Read the model definition and answer for the solid it produces. Units are mm, in the model's axes. A direction names the side the tool comes from. Round coordinates to 2 decimals unless told otherwise and drop trailing zeros. Write each loop counter-clockwise with the first axis right and the second up, starting at its lowest first coordinate (ties: lowest second). Pieces come first, ordered by that corner, then holes.
from build123d import *

# Parameters (mm, degrees)
SKETCH1_W           = 280
SKETCH1_H           = 210
BOSS_EXTRUDE1_DEPTH = 15
SKETCH2_R           = 5
BOSS_EXTRUDE2_DEPTH = 50
SKETCH3_W           = 10
SKETCH3_H           = 30
BOSS_EXTRUDE3_DEPTH = 50
SKETCH4_R           = 13
CUT_EXTRUDE1_DEPTH  = 20
SKETCH5_W           = 360.4909063
SKETCH5_H           = 249.182613404
SKETCH5_W_2         = 248.173776912
SKETCH5_H_2         = 125.095724948
CUT_EXTRUDE5_DEPTH  = 15
CUT_EXTRUDE6_START  = -65
SKETCH7_R           = 5
CUT_EXTRUDE6_DEPTH  = 65
SKETCH8_R           = 10.1
CUT_EXTRUDE11_DEPTH = 12
SKETCH13_W          = 26.98462743
SKETCH13_H          = 41.59552633
CUT_EXTRUDE12_DEPTH = 148.681383345
SKETCH11_W          = 17.231524428
SKETCH11_H          = 37.334969593
CUT_EXTRUDE13_DEPTH = 50
CUT_EXTRUDE16_DEPTH = 140.766916639
SKETCH16_R          = 13
CUT_EXTRUDE20_DEPTH = 5
CUT_EXTRUDE22_DEPTH = 2
SKETCH18_R          = 15.15
CUT_EXTRUDE23_DEPTH = 2
SKETCH9_W           = 29.33
SKETCH9_H           = 16.92
CUT_EXTRUDE24_DEPTH = 140.766916639


with BuildPart() as part:
    # Sketch1 → Boss-Extrude1 (new body)
    with BuildSketch(Plane(origin=(0, 0, 0), x_dir=(1, 0, 0), z_dir=(0, 1, 0))):
        Rectangle(SKETCH1_W, SKETCH1_H)
    extrude(amount=BOSS_EXTRUDE1_DEPTH)

    # Sketch2 → Boss-Extrude2 (add)
    with BuildSketch(Plane(origin=(0, 15, 0), x_dir=(1, 0, 0), z_dir=(0, 1, 0))):
        with Locations(Location((-100, 0, 0), (0, 0, 270))):
            Circle(SKETCH2_R)
        with Locations(Location((-100, 45, 0), (0, 0, 270))):
            Circle(SKETCH2_R)
        with Locations(Location((-100, -45, 0), (0, 0, 270))):
            Circle(SKETCH2_R)
    extrude(amount=BOSS_EXTRUDE2_DEPTH)

    # Sketch3 → Boss-Extrude3 (add)
    with BuildSketch(Plane(origin=(0, 15, 0), x_dir=(1, 0, 0), z_dir=(0, 1, 0))):
        Rectangle(SKETCH3_W, SKETCH3_H)
    extrude(amount=BOSS_EXTRUDE3_DEPTH)

    # Sketch4 → Cut-Extrude1 (cut)
    with BuildSketch(Plane(origin=(5, 0, 0), x_dir=(0, 0, -1), z_dir=(1, 0, 0))):
        with Locations((0, 41.236240869)):
            Circle(SKETCH4_R)
    extrude(amount=-CUT_EXTRUDE1_DEPTH, mode=Mode.SUBTRACT)

    # Sketch5 → Cut-Extrude5 (cut)
    with BuildSketch(Plane(origin=(0, 0, 0), x_dir=(1, 0, 0), z_dir=(0, 1, 0))):
        with Locations((1.345115322, -3.19464889)):
            Rectangle(SKETCH5_W, SKETCH5_H)
        Rectangle(SKETCH5_W_2, SKETCH5_H_2, mode=Mode.SUBTRACT)
    extrude(amount=CUT_EXTRUDE5_DEPTH, mode=Mode.SUBTRACT)

    # Sketch7 → Cut-Extrude6 (cut)
    with BuildSketch(Plane(origin=(0, 65, 0), x_dir=(1, 0, 0), z_dir=(0, 1, 0)).offset(CUT_EXTRUDE6_START)):
        with Locations(Location((-100, 45, 0), (0, 0, 270))):
            Circle(SKETCH7_R)
        with Locations(Location((-100, 0, 0), (0, 0, 270))):
            Circle(SKETCH7_R)
        with Locations(Location((-100, -45, 0), (0, 0, 270))):
            Circle(SKETCH7_R)
    extrude(amount=CUT_EXTRUDE6_DEPTH, mode=Mode.SUBTRACT)

    # Sketch8 → Cut-Extrude11 (cut)
    with BuildSketch(Plane.XZ):
        with Locations(Location((-100, 45, 0), (0, 0, 270))):
            Circle(SKETCH8_R)
        with Locations(Location((-100, 0, 0), (0, 0, 270))):
            Circle(SKETCH8_R)
        with Locations(Location((-100, -45, 0), (0, 0, 270))):
            Circle(SKETCH8_R)
    extrude(amount=-CUT_EXTRUDE11_DEPTH, mode=Mode.SUBTRACT)

    # Sketch13 → Cut-Extrude12 (cut, through all)
    with BuildSketch(Plane(origin=(0, 15, 0), x_dir=(1, 0, 0), z_dir=(0, 1, 0))):
        with Locations((-56.507686285, 0.099999998)):
            Rectangle(SKETCH13_W, SKETCH13_H)
    extrude(amount=-CUT_EXTRUDE12_DEPTH, mode=Mode.SUBTRACT)

    # Sketch11 → Cut-Extrude13 (cut)
    with BuildSketch(Plane(origin=(0, 65, 0), x_dir=(1, 0, 0), z_dir=(0, 1, 0))):
        with Locations((-3.002833284, 0.13632265)):
            Rectangle(SKETCH11_W, SKETCH11_H)
    extrude(amount=-CUT_EXTRUDE13_DEPTH, mode=Mode.SUBTRACT)

    # Sketch10 → Cut-Extrude16 (cut, through all)
    with BuildSketch(Plane(origin=(0, 15, 0), x_dir=(1, 0, 0), z_dir=(0, 1, 0))):
        Polygon((10.617962241, 13.651558309), (10.617962241, -16.40773575), (21.11227659, -7.629229077), (21.11227659, -32.023722987), (10.617962241, -26.348441691), (10.617962241, -56.40773575), (21.11227659, -47.629229077), (21.11227659, -62.347862477), (41.181983769, -80.61345612), (118.859305744, -85.146591928), (147.57727439, -51.586107965), (147.57727439, 65.118065893), (115.028872781, 75.532398006), (21.11227659, 80.76325418), (21.11227659, 62.347862473), (21.11227659, 47.976277013), (10.617962241, 53.651558309), (10.617962241, 23.59226425), (21.11227659, 32.370770923), (21.11227659, 7.976277013), align=None)
    extrude(amount=-CUT_EXTRUDE16_DEPTH, mode=Mode.SUBTRACT)

    # Sketch16 → Cut-Extrude20 (cut)
    with BuildSketch(Plane(origin=(0, 15, 0), x_dir=(1, 0, 0), z_dir=(0, 1, 0))):
        with Locations(Location((-100, 0, 0), (0, 0, 270))):
            Circle(SKETCH16_R)
    extrude(amount=-CUT_EXTRUDE20_DEPTH, mode=Mode.SUBTRACT)

    # Sketch17 → Cut-Extrude22 (cut)
    with BuildSketch(Plane.XZ):
        Polygon((-99.150124323, 10.064179616), (-99.150124323, 12.064179616), (-100.650124323, 12.064179616), (-100.650124323, 10.064179616), (-100.726397945, 9.213176312), (-99.150124323, 9.422776077), align=None)
    extrude(amount=-CUT_EXTRUDE22_DEPTH, mode=Mode.SUBTRACT)

    # Sketch18 → Cut-Extrude23 (cut)
    with BuildSketch(Plane(origin=(0, 15, 0), x_dir=(1, 0, 0), z_dir=(0, 1, 0))):
        with Locations(Location((-100, 0, 0), (0, 0, 270))):
            Circle(SKETCH18_R)
    extrude(amount=-CUT_EXTRUDE23_DEPTH, mode=Mode.SUBTRACT)

    # Sketch9 → Cut-Extrude24 (cut, through all)
    with BuildSketch(Plane(origin=(0, 15, 0), x_dir=(1, 0, 0), z_dir=(0, 1, 0))):
        with Locations((-19.421888456, 47.087862474)):
            Rectangle(SKETCH9_W, SKETCH9_H)
    extrude(amount=-CUT_EXTRUDE24_DEPTH, mode=Mode.SUBTRACT)


solid = part.part
Q1. Section D-D (x = -55) is taken. Determine the outline of the cut face in (y, z), then the cut area to 3 significant figures.
Verdict:
outline: (0, -62.55) - (15, -62.55) - (15, -20.9) - (0, -20.9) - close; (0, 20.7) - (15, 20.7) - (15, 62.55) - (0, 62.55) - close
area: 1,250 mm2
Q2. Flat-ended cylindrical pins translate along their axes: pin 1 Ø6 at (x, z) = (-9, 39.5) entering from -Y; pin 2 Ø7.5 at (y, z) = (7, 44.5) entering from +X; pin 3 Ø13 at (x, z) = (-100, 45) entering from -Y; pin 4 Ø7.5 at (y, z) = (6, -37) entering from +X. Find the tip coordinate at first contact, or state that the pin passes through.
Verdict:
pin 1: stops at y = 0
pin 2: stops at x = 21.11
pin 3: stops at y = 12
pin 4: stops at x = 10.62
Q3. Section B-B (y = 6.25) is taken. Determine the outline of the cut face in (x, z).
Verdict:
outline: (-124.09, -62.55) - (21.11, -62.55) - (21.11, -47.98) - (10.62, -53.65) - (10.62, -23.59) - (21.11, -32.37) - (21.11, -7.98) - (10.62, -13.65) - (10.62, 16.41) - (21.11, 7.63) - (21.11, 32.02) - (10.62, 26.35) - (10.62, 56.41) - (21.11, 47.63) - (21.11, 62.35) - (21.33, 62.55) - (-124.09, 62.55) - close; hole circle Ø20.2 at (-100, -45); hole circle Ø20.2 at (-100, 0); hole circle Ø20.2 at (-100, 45); hole (-70, -20.9) - (-43.02, -20.9) - (-43.02, 20.7) - (-70, 20.7) - close; hole (-34.09, -55.55) - (-4.76, -55.55) - (-4.76, -38.63) - (-34.09, -38.63) - close
Q4. Section A-A (z = -45) is taken. Determine the outline of the cut face in (x, y).
Verdict:
outline: (-124.09, 0) - (-110.1, 0) - (-110.1, 12) - (-105, 12) - (-105, 15) - (-124.09, 15) - close; (-95, 12) - (-89.9, 12) - (-89.9, 0) - (-34.09, 0) - (-34.09, 15) - (-95, 15) - close; (-4.76, 0) - (10.62, 0) - (10.62, 15) - (-4.76, 15) - close
Q5. Section C-C (z = 45) is taken. Determine the outline of the cut face in (x, y).
Verdict:
outline: (-124.09, 0) - (-110.1, 0) - (-110.1, 12) - (-105, 12) - (-105, 15) - (-124.09, 15) - close; (-95, 12) - (-89.9, 12) - (-89.9, 0) - (10.62, 0) - (10.62, 15) - (-95, 15) - close
Q6. Which of the six approach directions +Z, -Z, +X, -X, +Y, -Y give full straight-line access (tool end or side, diameter ignored) to faces 1 (the flat face through (-95, 12, -47)), 2 (the cylindrical face through (-112.69, 11.52, -2.82)), 3 (the flat face through (15.79, 7.6, 52.08)), 4 (the flat face through (21.112, 8, -20))?
Verdict:
face 1: -Y
face 2: +Y
face 3: +Y, -Y
face 4: -Z, +X, +Y, -Y
Q7. Straight lines are drawn through the part: probe 1 along X at (y, z) = (7, -45); probe 2 along X at (y, z) = (7.25, 0); probe 3 along Z at (x, y) = (-56, 14.25). For each, find the intervals that lie inside material, in ascending order.
Verdict:
probe 1: x = -124.09 to -110.1, -89.9 to -34.09, -4.76 to 10.62
probe 2: x = -124.09 to -110.1, -89.9 to -70, -43.02 to 10.62
probe 3: z = -62.55 to -20.9, 20.7 to 62.55
Q8. Determine the mould class of faces 5 (the flat face through (10.618, 8, -39)), 6 (the flat face through (21.112, 8, 20)), 7 (the flat face through (-52, 7, 62.548)) for opening direction Z: pulls with the +Z half, pulls with the -Z half, needs draft (parallel to the pull), parting line crosses it, or undercut.
Verdict:
face 5: undercut
face 6: needs draft
face 7: pulls with the +Z half
